Part model, mm, in its own coordinate system. Face numbers are marked on the shaded views. Round coordinates to 2 decimals unless told otherwise and drop trailing zeros. Loops run counter-clockwise (first coordinate to the right, second up) from the corner with the lowest first, then second, coordinate; pieces in that order, holes last. Notation, with made-up numbers: (77.25, 22) -> (91.25, 22) arc R14 cw to (91.25, 36) -> close; hole circle Ø8 at (60, 38.5). An arc over 180 degrees is marked (long way). Answer as a JSON object with one key per item and string values. Group by question number.
from build123d import *

# Parameters (mm, degrees)
BOSS_EXTRUDE1_DEPTH        = 2.6
SKETCH5_W                  = 11.826356456
SKETCH5_H                  = 5.621169426
CUT_EXTRUDE2_DEPTH         = 1.105635064
SKETCH6_W                  = 11.690711404
SKETCH6_H                  = 7.254613366
CUT_EXTRUDE3_DEPTH         = 5.2
BOSS_EXTRUDE2_START        = -0.052804
SKETCH7_R                  = 0.353553391
BOSS_EXTRUDE2_DEPTH        = 12.752804
SKETCH8_R                  = 0.8
CUT_EXTRUDE4_DEPTH         = 0.2
CROQUIS1_W                 = 6.923561314
CROQUIS1_H                 = 11.497610845
CORTAR_EXTRUIR1_DEPTH      = 5
CORTAR_EXTRUIR1_DEPTH_BACK = 5


with BuildPart() as part:
    # Sketch2 → Boss-Extrude1 (new body, symmetric)
    with BuildSketch(Plane(origin=(0, 0, 0), x_dir=(1, 0, 0), z_dir=(0, 1, 0))):
        with BuildLine():
            Line((-2.105447518, 1.212026432), (2.105447518, 1.212026432))
            ThreePointArc((2.105447518, 1.212026432), (0, -2.977973568), (-2.105447518, 1.212026432))
        make_face()
    extrude(amount=BOSS_EXTRUDE1_DEPTH, both=True)

    # Sketch5 → Cut-Extrude2 (cut, through all)
    with BuildSketch(Plane(origin=(0, 2.580250079, -0.225742631), x_dir=(1, 0, 0), z_dir=(0, 0.996194698, -0.087155743))):
        with Locations((0.924694538, -0.744658901)):
            Rectangle(SKETCH5_W, SKETCH5_H)
    cut_extrude2 = extrude(amount=CUT_EXTRUDE2_DEPTH, mode=Mode.SUBTRACT)

    # Sketch6 → Cut-Extrude3 (cut)
    with BuildSketch(Plane(origin=(0, 2.580250079, 0.225742631), x_dir=(1, 0, 0), z_dir=(0, 0.996194698, 0.087155743))):
        with Locations((0.257342704, -2.465539164)):
            Rectangle(SKETCH6_W, SKETCH6_H)
    cut_extrude3 = extrude(amount=CUT_EXTRUDE3_DEPTH, mode=Mode.SUBTRACT)

    # Mirror1: Cut-Extrude2, Cut-Extrude3 across plane
    add(cut_extrude2.mirror(Plane.ZX), mode=Mode.SUBTRACT)
    add(cut_extrude3.mirror(Plane.ZX), mode=Mode.SUBTRACT)

    # Sketch7 → Boss-Extrude2 (add)
    with BuildSketch(Plane(origin=(0, -2.6, 0), x_dir=(-1, 0, 0), z_dir=(0, -1, 0)).offset(BOSS_EXTRUDE2_START)):
        with Locations((-1.27, 0.25)):
            Circle(SKETCH7_R)
        with Locations((0, 0.25)):
            Circle(SKETCH7_R)
        with Locations((1.27, 0.25)):
            Circle(SKETCH7_R)
    extrude(amount=BOSS_EXTRUDE2_DEPTH)

    # Sketch8 → Cut-Extrude4 (cut)
    with BuildSketch(Plane.XY.offset(2.977973568)):
        Circle(SKETCH8_R)
    extrude(amount=-CUT_EXTRUDE4_DEPTH, mode=Mode.SUBTRACT)

    # Croquis1 → Cortar-Extruir1 (cut, two sides)
    with BuildSketch(Plane(origin=(0, 0, 0), x_dir=(0, 0, -1), z_dir=(1, 0, 0))) as cortar_extruir1_sk:
        with Locations((0.104321276, -10.336671587)):
            Rectangle(CROQUIS1_W, CROQUIS1_H)
    extrude(amount=CORTAR_EXTRUIR1_DEPTH, mode=Mode.SUBTRACT)
    extrude(cortar_extruir1_sk.sketch, amount=-CORTAR_EXTRUIR1_DEPTH_BACK, mode=Mode.SUBTRACT)


solid = part.part
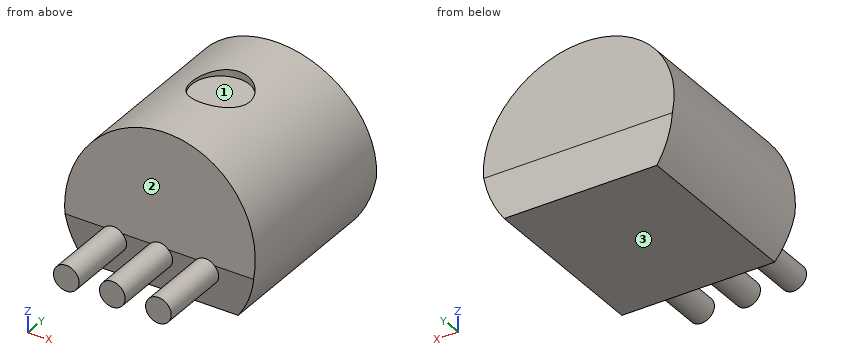
Item 1: Band-saw the part on B-B, the plane y = -3.25. List the corners of the cut face in (x, z), plus the area to 3 significant figures.
Item 2: Band-saw the part on A-A, the plane x = 0.55. List the corners of the cut face in (y, z).
Item 3: Band-saw the part on C-C, the plane z = -0.25. List the corners of the cut face in (x, y), plus the area to 3 significant figures.
Item 4: Two-plate mould, pull along Y, no slides. Class the marked faces 1, 2 and 3: pulls with the +Y half, pulls with the -Y half, needs draft (parallel to the pull), parting line crosses it, or undercut.
Item 5: Band-saw the part on D-D, the plane y = 0. List the corners of the cut face in (x, z).
Item 6: Drill centre lines: line 1 (Y direction, x = 0, z = 2.9); line 2 (Y direction, x = 1, z = -0.4) (3 decimals); line 3 (Y direction, x = -0.8, z = -0.35). Where is each one in solid material? Low to high.
Item 7: Drop flat-ended pins along their axis: pin 1 Ø1.3 at (x, y) = (0, 0) entering from +Z; pin 2 Ø3 at (x, y) = (1.5, 1) entering from +Z; pin 3 Ø1 at (x, y) = (1, 0.5) entering from +Z. Give the stop position or say it passes through.
Entries:
{
 "1": {"outline": "circle Ø0.71 at (-1.27, -0.25); circle Ø0.71 at (0, -0.25); circle Ø0.71 at (1.27, -0.25)", "area": "1.18 mm²"},
 "2": {"outline": "(-2.6, 0) -> (-2.49, -1.21) -> (2.49, -1.21) -> (2.6, 0) -> (2.34, 2.92) -> (0.58, 2.92) -> (0.58, 2.78) -> (-0.58, 2.78) -> (-0.58, 2.92) -> (-2.34, 2.92) -> close"},
 "3": {"outline": "(-2.55, -2.58) -> (-1.62, -2.58) -> (-1.62, -4.59) -> (-0.92, -4.59) -> (-0.92, -2.58) -> (-0.35, -2.58) -> (-0.35, -4.59) -> (0.35, -4.59) -> (0.35, -2.58) -> (0.92, -2.58) -> (0.92, -4.59) -> (1.62, -4.59) -> (1.62, -2.58) -> (2.55, -2.58) -> (2.55, 2.58) -> (-2.55, 2.58) -> close", "area": "30.6 mm²"},
 "4": {"face 1": "undercut", "face 2": "pulls with the -Y half", "face 3": "needs draft"},
 "5": {"outline": "(-2.11, -1.21) -> (2.11, -1.21) arc R2.62 ccw to (0.8, 2.85) -> (0.8, 2.78) -> (-0.8, 2.78) -> (-0.8, 2.85) arc R2.62 ccw to start"},
 "6": {"line 1": "-2.35 to -0.8, 0.8 to 2.35", "line 2": "-4.588 to 2.565", "line 3": "-2.57 to 2.57"},
 "7": {"pin 1": "z = 2.78", "pin 2": "z = 2.98", "pin 3": "z = 2.93"}
}
